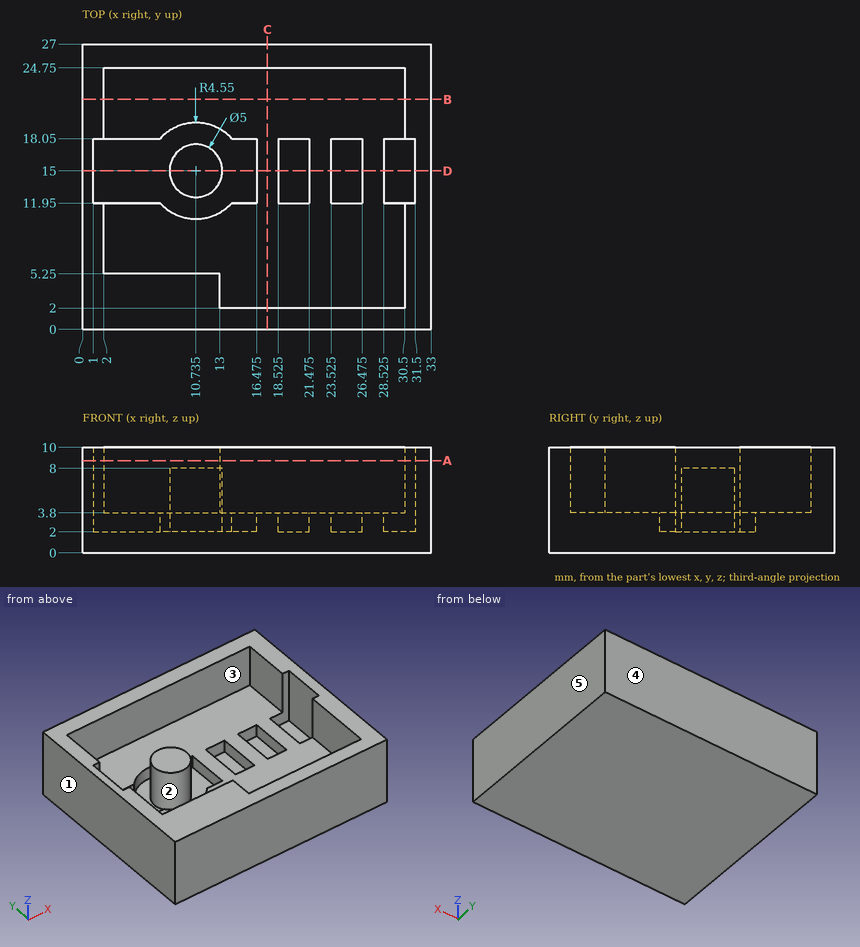
Check sheet for the drawn part. Datum: minimum x, y, z corner. Units: mm. A direction names the side the tool comes from. Coordinates: 2 decimals unless noted, no trailing zeros. Order: outer loops, then holes, each group sorted by start corner. A loop starts at its lowest first (then second) coordinate and runs counter-clockwise, first axis right, second up. Notation, with made-up numbers: M 64.25,57.5 L 88.25,57.5 A7 cw 88.25,70.5 Z; hole C 33.25,63.25 d8. An arc over 180 degrees is marked long. One line per item, written item: value. Start each with the question number.
Item 1: Mould release check, pull along Y, two halves, no side actions. Record for the marked faces 3, 4 and 5: released by +Y, released by -Y, zero draft, split by the parting line, or undercut.
Item 2: Sectioned sample at A-A (z = 8.75). Enter the section's corners in (x, y), then the cut area to 3 significant figures.
Item 3: Scan lines: probe 1 along Y at (x, z) = (16, 4.25); probe 2 along Y at (x, z) = (11, 9); probe 3 along X at (y, z) = (9.25, 9.75). Record each from-to range of solid material in increasing order.
Item 4: Gauge pin test, flat ends, axial feed: pin 1 (4 mm diameter, centred on x = 11, y = 14, fed in from +Z); pin 2 (4 mm diameter, centred on x = 25, y = 21.5, fed in from +Z); pin 3 (1.5 mm diameter, centred on x = 30, y = 16, fed in from +Z). Record the tip position at first contact, or that the pin passes through.
Item 5: Sectioned sample at B-B (y = 21.75). Enter the section's corners in (x, z), then the cut area to 3 significant figures.
Item 6: Sectioned sample at D-D (y = 15). Enter the section's corners in (x, z) (3 decimals).
Item 7: Access from +Z, -Z, +X, -X, +Y, -Y to the whole of each face (thin tool, end or side, straight path). Record for the marked faces 1 and 2.
Item 8: Sectioned sample at C-C (x = 17.5). Enter the section's corners in (y, z).
Conclusion:
1. face 3: undercut
1. face 4: released by +Y
1. face 5: zero draft
2. outline: M 0,0 L 33,0 L 33,27 L 0,27 Z; hole M 1,11.95 L 2,11.95 L 2,5.25 L 13,5.25 L 13,2 L 30.5,2 L 30.5,11.95 L 31.5,11.95 L 31.5,18.05 L 30.5,18.05 L 30.5,24.75 L 2,24.75 L 2,18.05 L 1,18.05 Z
2. area: 266 mm^2
3. probe 1: y = 0 to 2, 24.75 to 27
3. probe 2: y = 0 to 5.25, 24.75 to 27
3. probe 3: x = 0 to 2, 30.5 to 33
4. pin 1: stops at z = 8
4. pin 2: stops at z = 3.8
4. pin 3: stops at z = 2
5. outline: M 0,0 L 33,0 L 33,10 L 30.5,10 L 30.5,3.8 L 2,3.8 L 2,10 L 0,10 Z
5. area: 153 mm^2
6. outline: M 0,0 L 33,0 L 33,10 L 31.5,10 L 31.5,2 L 28.525,2 L 28.525,3.8 L 26.475,3.8 L 26.475,2 L 23.525,2 L 23.525,3.8 L 21.475,3.8 L 21.475,2 L 18.525,2 L 18.525,3.8 L 16.475,3.8 L 16.475,2 L 13.235,2 L 13.235,8 L 8.235,8 L 8.235,2 L 1,2 L 1,10 L 0,10 Z
7. face 1: +Z, -Z, -X, +Y, -Y
7. face 2: +Z
8. outline: M 0,0 L 27,0 L 27,10 L 24.75,10 L 24.75,3.8 L 2,3.8 L 2,10 L 0,10 Z
